from build123d import *

# Parameters (mm, degrees)
SKETCH_1_W          = 38
SKETCH_1_H          = 12
EXTRUDE_1_DEPTH     = 1.2
SKETCH_2_W          = 30
SKETCH_2_H          = 11
EXTRUDE_2_DEPTH     = 2.7
SKETCH_3_R          = 0.75
CUT_EXTRUDE_2_DEPTH = 39.565399
EXTRUDE_START       = 1.2
SKETCH_4_W          = 2
SKETCH_4_H          = 10
SKETCH_4_H_2        = 1.370131764
EXTRUDE_3_DEPTH     = 2


with BuildPart() as part:
    # Эскиз1 → Бобышка-Вытянуть1 (new body)
    with BuildSketch(Plane(origin=(0, 0, 0), x_dir=(1, 0, 0), z_dir=(0, 1, 0))):
        with Locations((-19, 0)):
            Rectangle(SKETCH_1_W, SKETCH_1_H)
    extrude(amount=EXTRUDE_1_DEPTH)

    # Эскиз2 → Бобышка-Вытянуть2 (add)
    with BuildSketch(Plane(origin=(0, 0, 0), x_dir=(1, 0, 0), z_dir=(0, 1, 0))):
        with Locations((-20, 0)):
            Rectangle(SKETCH_2_W, SKETCH_2_H)
    extrude(amount=EXTRUDE_2_DEPTH)

    # Эскиз3 → Вырез-Вытянуть2 (cut, through all)
    with BuildSketch(Plane(origin=(0, 0, 0), x_dir=(1, 0, 0), z_dir=(0, 1, 0))):
        with Locations(Location((-2, 4, 0), (0, 0, 90))):
            Circle(SKETCH_3_R)
        with Locations(Location((-2, 1.333333333, 0), (0, 0, 90))):
            Circle(SKETCH_3_R)
        with Locations(Location((-2, -1.333333333, 0), (0, 0, 90))):
            Circle(SKETCH_3_R)
        with Locations(Location((-2, -4, 0), (0, 0, 90))):
            Circle(SKETCH_3_R)
    extrude(amount=CUT_EXTRUDE_2_DEPTH, mode=Mode.SUBTRACT)

    # Эскиз4 → Бобышка-Вытянуть3 (add)
    with BuildSketch(Plane(origin=(0, 0, 0), x_dir=(1, 0, 0), z_dir=(0, 1, 0)).offset(EXTRUDE_START)):
        with Locations((-23, 0)):
            Rectangle(SKETCH_4_W, SKETCH_4_H)
        with Locations((-16, 0)):
            Rectangle(SKETCH_4_W, SKETCH_4_H)
        with Locations((-10.327262123, 1.918184469)):
            Rectangle(SKETCH_4_W, SKETCH_4_H_2)
    extrude(amount=-EXTRUDE_3_DEPTH)


solid = part.part
Read the model definition and answer for the solid it produces. Units are mm, in the model's axes. A direction names the side the tool comes from. Coordinates: 2 decimals unless noted, no trailing zeros. Loops run counter-clockwise (first coordinate to the right, second up) from the corner with the lowest first, then second, coordinate; pieces in that order, holes last. Notation, with made-up numbers: (-30, 43.5) -> (27, 43.5) arc R22 cw to (27, 49.5) -> close; hole circle Ø8 at (-38.75, 35.25). An arc over 180 degrees is marked (long way). Write item = value, one per line. Start each with the question number.
1) The part is cut by section D-D, the plane x = -13. Determine the outline of the cut face in (y, z).
2) The part is cut by section B-B, the plane z = 4. Determine the outline of the cut face in (x, y), plus the area to 3 significant figures.
3) The part is cut by section C-C, the plane x = -2. Determine the outline of the cut face in (y, z), plus the area to 3 significant figures.
4) Find the intervals of material crossed by L1, parallel to X at y = 0.6, z = 4; L2, parallel to X at y = -0.4, z = -3.5; L3, parallel to Y at x = -34.5, z = 3, in increasing order. Write a range as from..to.
5) The mould has two halves that part along X. Classify faces 4 (the face through (-2.033, 0.592, 2.083)), 5 (the face through (0, 1, 0)), 6 (the face through (-19, 1, -6)): pulls with the +X half, pulls with the -X half, needs draft (parallel to the pull), parting line crosses it, or undercut.
6) The part is cut by section A-A, the plane y = 0.55. Determine the outline of the cut face in (x, z).
7) For faces 1 (the face through (-20, 2, -5.5)), 2 (the face through (-35, 2, 0)), 3 (the face through (-20, 2, 5.5)), determine the directions among +Z, -Z, +X, -X, +Y, -Y from which every point of the face is accessible in a straight line to the end or side of a thin tool.
8) Given P1, Ø1, axis at x = -24.5, y = 2, coming from the +Z side; P2, Ø1.5, axis at x = -19.5, z = -4, coming from the -Y side; P3, Ø0.6, axis at y = -0.5, z = -0.5, coming from the +X side, each flat-ended and moving along its own axis, determine where each tip first touches the part or whether it passes through.
Result:
q1.outline = (0, -6) -> (1.2, -6) -> (1.2, -5.5) -> (2.7, -5.5) -> (2.7, 5.5) -> (1.2, 5.5) -> (1.2, 6) -> (0, 6) -> close
q2.outline = (-38, 0) -> (-24, 0) -> (-24, -0.8) -> (-22, -0.8) -> (-22, 0) -> (-17, 0) -> (-17, -0.8) -> (-15, -0.8) -> (-15, 0) -> (-2.75, 0) -> (-2.75, 1.2) -> (-5, 1.2) -> (-5, 2.7) -> (-35, 2.7) -> (-35, 1.2) -> (-38, 1.2) -> close; (-1.25, 0) -> (0, 0) -> (0, 1.2) -> (-1.25, 1.2) -> close
q2.area = 92.0 mm²
q3.outline = (0, -6) -> (1.2, -6) -> (1.2, -4.75) -> (0, -4.75) -> close; (0, -3.25) -> (1.2, -3.25) -> (1.2, -2.08) -> (0, -2.08) -> close; (0, -0.58) -> (1.2, -0.58) -> (1.2, 0.58) -> (0, 0.58) -> close; (0, 2.08) -> (1.2, 2.08) -> (1.2, 3.25) -> (0, 3.25) -> close; (0, 4.75) -> (1.2, 4.75) -> (1.2, 6) -> (0, 6) -> close
q3.area = 7.20 mm²
q4.L1 = -38..-2.75, -1.25..0
q4.L2 = -24..-22, -17..-15
q4.L3 = 0..2.7
q5.face_4 = undercut
q5.face_5 = pulls with the +X half
q5.face_6 = needs draft
q6.outline = (-38, -6) -> (0, -6) -> (0, 6) -> (-38, 6) -> close; hole circle Ø1.5 at (-2, -4); hole circle Ø1.5 at (-2, -1.33); hole circle Ø1.5 at (-2, 1.33); hole circle Ø1.5 at (-2, 4)
q7.face_1 = -Z, +X, -X, +Y
q7.face_2 = +Z, -Z, -X, +Y
q7.face_3 = +Z, +X, -X, +Y
q8.P1 = 5.5
q8.P2 = 0
q8.P3 = -15
